The figure shows three views and two pictorial views of one solid part (mm, origin at its lowest corner). Answer the questions. A direction names the side the tool comes from. Round coordinates to 2 decimals unless told otherwise and drop trailing zeros. Order: outer loops, then holes, each group sorted by start corner. A loop starts at its lowest first (then second) coordinate and runs counter-clockwise, first axis right, second up. Notation, with made-up numbers: M 44,-36.5 L 49,-36.5 A28 ccw 49,0.5 Z; hole C -18.75,3.5 d4. An arc over 180 degrees is marked long. Answer as CSV lines item,"result".
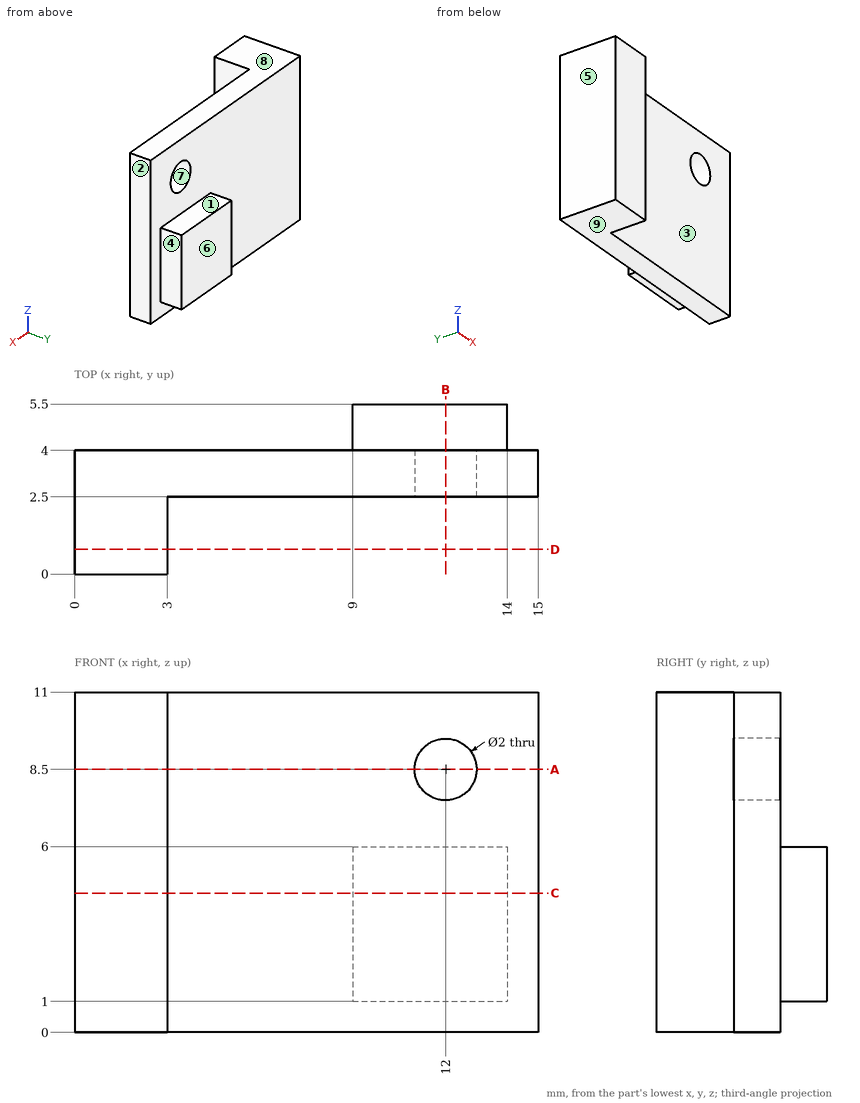
Item 1: Determine the mould class of the marked faces 6, 7, 8 and 9 for opening direction Z: +Z half, -Z half, draft (parallel to the pull), parting line (faces both ways), or undercut.
Ans:
face 6,"draft"
face 7,"undercut"
face 8,"+Z half"
face 9,"-Z half"
Item 2: A cutting plane is placed at A-A, the plane z = 8.5. Determine the outline of the cut face in (x, y).
Ans:
outline,"M 0,0 L 3,0 L 3,2.5 L 11,2.5 L 11,4 L 0,4 Z; M 13,2.5 L 15,2.5 L 15,4 L 13,4 Z"
Item 3: Flat-ended cylindrical pins translate along their axes: pin 1 (0.8 mm diameter, centred on y = 1, z = 6, fed in from +X); pin 2 (1.6 mm diameter, centred on x = 10.5, y = 5, fed in from +Z); pin 3 (5.5 mm diameter, centred on x = 9, z = 7.5, fed in from -Y). Find the tip coordinate at first contact, or state that the pin passes through.
Ans:
pin 1,"x = 3"
pin 2,"z = 6"
pin 3,"y = 2.5"
Item 4: A cutting plane is placed at C-C, the plane z = 4.5. Determine the outline of the cut face in (x, y), and give its area (3 significant figures).
Ans:
outline,"M 0,0 L 3,0 L 3,2.5 L 15,2.5 L 15,4 L 14,4 L 14,5.5 L 9,5.5 L 9,4 L 0,4 Z"
area,"37.5 mm2"
Item 5: A cutting plane is placed at D-D, the plane y = 0.8. Determine the outline of the cut face in (x, z).
Ans:
outline,"M 0,0 L 3,0 L 3,11 L 0,11 Z"
Item 6: A tool of negligible diameter and unlimited length cuts with its end or side. For the marked faces 1, 2, 3, 4 and 5, from which of +Z, -Z, +X, -X, +Y, -Y can it reach the whole face along a straight path? Write none if from no direction.
Ans:
face 1,"+Z, +X, -X, +Y"
face 2,"+Z, -Z, +X, +Y, -Y"
face 3,"+Z, -Z, +X, -Y"
face 4,"+Z, -Z, +X, +Y"
face 5,"+Z, -Z, -X, +Y, -Y"
Item 7: Find the intervals of material crossed by probe 1 along X at (y, z) = (3.2, 8.5); probe 2 along Z at (x, y) = (12, 3); probe 3 along Y at (x, z) = (6.5, 7.25), in increasing order. Write a range as [from, to].
Ans:
probe 1,"[0, 11], [13, 15]"
probe 2,"[0, 7.5], [9.5, 11]"
probe 3,"[2.5, 4]"
Item 8: A cutting plane is placed at B-B, the plane x = 12. Determine the outline of the cut face in (y, z).
Ans:
outline,"M 2.5,0 L 4,0 L 4,1 L 5.5,1 L 5.5,6 L 4,6 L 4,7.5 L 2.5,7.5 Z; M 2.5,9.5 L 4,9.5 L 4,11 L 2.5,11 Z"
